Build history of the part. All positions in model axes, mm. Round coordinates to 2 decimals unless told otherwise and drop trailing zeros. Write each loop counter-clockwise with the first axis right and the second up, starting at its lowest first coordinate (ties: lowest second). Pieces come first, ordered by that corner, then holes. Notation, with made-up numbers: (31, 70) - (87, 70) arc R35 cw to (87, 102) - close; hole circle Ø2 at (85.25, -34.5). An arc over 180 degrees is marked (long way). Write each question's results on one line, items separated by ' | '.
Autodesk Inventor part; units mm, degrees
ref_plane "YZ Plane" through (0, 0, 0) normal (1, 0, 0) x (0, 1, 0)
ref_plane "XZ Plane" through (0, 0, 0) normal (0, 1, 0) x (-1, 0, 0)
ref_plane "XY Plane" through (0, 0, 0) normal (0, 0, 1) x (1, 0, 0)
sketch "Sketch1" plane through (0, 0, 0) normal (0, 1, 0) x (-1, 0, 0)
  line L0 (-3.175, -3.175) -> (3.175, -3.175)
  line L1 (3.175, -3.175) -> (3.175, 3.175)
  line L2 (3.175, 3.175) -> (-3.175, 3.175)
  line L3 (-3.175, 3.175) -> (-3.175, -3.175)
  line L4 (-3.175, -3.175) -> (3.175, 3.175) construction
  line L5 (3.175, -3.175) -> (-3.175, 3.175) construction
  point P0 (0, 0)
  dimension "d0" = 6.35
  dimension "d1" = 6.35
extrude "Extrusion1" add sketch "Sketch1" along normal blind 330.2
fillet "Fillet1" radius 1.5875 4 edges at (-3.175, 165.1, -3.175) (3.175, 165.1, -3.175) (3.175, 165.1, 3.175) (-3.175, 165.1, 3.175)
fillet "Fillet2" radius 0.7937 16 edges at (3.175, 0, 0) (2.71, 0, -2.71) (0, 0, -3.175) (-2.71, 0, -2.71) (-3.175, 0, 0) (-2.71, 0, 2.71) (0, 0, 3.175) (2.71, 0, 2.71) (0, 330.2, -3.175) (2.71, 330.2, -2.71) (3.175, 330.2, 0) (2.71, 330.2, 2.71) (0, 330.2, 3.175) (-2.71, 330.2, 2.71) (-3.175, 330.2, 0) (-2.71, 330.2, -2.71)
ref_plane "Work Plane1" through (0, 165.1, 0) normal (0, 1, 0) x (1, 0, 0)
properties part number "13in hs shaft" material "Stainless Steel"
(1) Slice it at A-A, the plane y = 159.5. Write the cut outline in (x, z) (1 decimal).
Worked answers:
outline: (-3.2, -1.6) arc R1.6 ccw to (-1.6, -3.2) - (1.6, -3.2) arc R1.6 ccw to (3.2, -1.6) - (3.2, 1.6) arc R1.6 ccw to (1.6, 3.2) - (-1.6, 3.2) arc R1.6 ccw to (-3.2, 1.6) - close
(2) Drill centre lines: probe 1 along Z at (x, y) = (1.75, 316.5); probe 2 along X at (y, z) = (72, 2). Where is each one in solid material? Low to high. Write a range as [from, to].
Worked answers:
probe 1: z = [-3.17, 3.17] | probe 2: x = [-3.12, 3.12]
(3) Flat gauge pin, fed straight in: pin 1 Ø3 at (x, z) = (2, 2.5) entering from +Y. Where does the tip first touch, or does it go through?
Worked answers:
pin 1: stops at y = 330.2
